from build123d import *

# Parameters (mm, degrees)
BOSS_EXTRUDE1_DEPTH = 5
FILLET1_R           = 2
FILLET2_R           = 1


with BuildPart() as part:
    # Sketch1 → Boss-Extrude1 (new body)
    with BuildSketch(Plane.XY):
        with BuildLine():
            Line((45.947382797642085, 2), (-124.5, 1.9999999999999962))
            Line((-124.5, 1.9999999999999962), (-124.5, 20.99999999999999))
            Line((-124.5, 20.99999999999999), (-109.6965869966638, 20.999999999999993))
            Line((-109.6965869966638, 20.999999999999993), (-109.6965869966638, 22.99999999999999))
            Line((-109.6965869966638, 22.99999999999999), (-126.5, 22.99999999999999))
            Line((-126.5, 22.99999999999999), (-126.5, -3.98e-15))
            Line((-126.5, -3.98e-15), (-96.00000000000003, -5.01e-15))
            ThreePointArc((-96.00000000000003, -1.3922e-13), (-91.91634498174992, -12.422936572760829), (-81.25831039658792, -19.999999999999993))
            Line((-81.25831039658792, -19.999999999999996), (-67.7416896034121, -19.999999999999996))
            ThreePointArc((-67.7416896034121, -20), (-59.22674645064795, -14.898875979359843), (-54.01801901082011, -6.449326782725662))
            ThreePointArc((-54.01801901082044, -6.449326782725638), (-49.745600463821845, -19.747926884371328), (-41.46929842095424, -31.000000000000007))
            Line((-41.46929842095423, -31), (-13.530701579045768, -31))
            ThreePointArc((-13.530701579045765, -31.000000000000004), (-5.5615533236631265, -20.33765705801185), (-1.1997684126617827, -7.76118245981885))
            ThreePointArc((-1.1997684126617756, -7.761182459818851), (1.6903832669508674, -16.34383705889386), (6.527542114603506, -24))
            Line((6.527542114603509, -24), (37.47245788539651, -24))
            ThreePointArc((37.47245788539651, -24), (44.12729350691807, -11.787963694678155), (45.947382797642085, 2))
        make_face()
        with BuildLine():
            ThreePointArc((-55.000000000000014, -3.1e-16), (-58.606442943263986, -11.117096597214955), (-68.05217786452643, -18))
            Line((-68.05217786452643, -18), (-80.94782213547359, -18))
            ThreePointArc((-80.94782213547359, -18.000000000000004), (-90.39355705673603, -11.117096597214955), (-94, -5.08e-15))
            Line((-94, -5.08e-15), (-55.00000000000001, -3.1e-16))
        make_face(mode=Mode.SUBTRACT)
        with BuildLine():
            ThreePointArc((-2.499999999999993, 0), (-5.579078670022007, -15.665382277262486), (-14.358195797467605, -28.999999999999996))
            Line((-14.358195797467618, -29), (-40.641804202532384, -29))
            ThreePointArc((-40.641804202532384, -29), (-49.420921329978, -15.665382277262491), (-52.500000000000014, 0))
            Line((-52.50000000000001, 0), (-2.5, 0))
        make_face(mode=Mode.SUBTRACT)
        with BuildLine():
            ThreePointArc((7.494737611193308, -21.999999999999993), (1.9251046025075595, -11.620790548201041), (0, 0))
            Line((0, 0), (44, 0))
            ThreePointArc((44, 0), (42.07489539749246, -11.620790548201052), (36.5052623888067, -22))
            Line((36.50526238880669, -22), (7.494737611193305, -21.999999999999986))
        make_face(mode=Mode.SUBTRACT)
    extrude(amount=BOSS_EXTRUDE1_DEPTH)

    # Fillet1
    # the kernel refuses this fillet: 2 mm, written as the material it adds along each edge
    with BuildSketch(Plane(origin=(7.494737611193306, -21.99999999999999, 0), x_dir=(-0.5991062369957058, 0.8006695428157894, 0), z_dir=(0, 0, 1))) as fillet1_piece_1:
        with BuildLine():
            CenterArc((1.0015491764552975, -1.9997957036664622), FILLET1_R, 89.18105145509278, 54.01303517716653)
            Line((-0.5997899091731567, -0.8015832296708748), (0, 0))
            ThreePointArc((0, 0), (0.5150674500576004, 0.00368108195627573), (1.030134900115199, -5e-17))
        make_face()
    extrude(amount=5)
    with BuildSketch(Plane(origin=(36.5052623888067, -22, 0), x_dir=(0.599106236995708, 0.8006695428157878, 0), z_dir=(0, 0, 1))) as fillet1_piece_2:
        with BuildLine():
            CenterArc((1.0015491764552726, 1.9997957036664615), FILLET1_R, 216.80591336773654, 54.01303517717065)
            Line((-0.5997899091732678, 0.8015832296709893), (0, 0))
            ThreePointArc((0, 0), (0.5150674500575887, -0.00368108195627645), (1.0301349001151745, 4e-17))
        make_face()
    extrude(amount=5)
    with BuildSketch(Plane(origin=(-1.1997684126617827, -7.7611824598188495, 0), x_dir=(-0.2559607440844839, -0.9666871766438806, 0), z_dir=(0, 0, 1))) as fillet1_piece_3:
        with BuildLine():
            CenterArc((7.006516264382127, 1.9937618524445377), FILLET1_R, 126.90247774602503, 138.57101311365483)
            ThreePointArc((5.80560665040515, 3.593079237786693), (2.9835854859434217, 1.6660138445939616), (0, 0))
            ThreePointArc((0, 0), (3.424337799359584, 0.13533600091225512), (6.84867559871917, -3e-17))
        make_face()
    extrude(amount=5)
    with BuildSketch(Plane(origin=(-14.358195797467612, -29, 0), x_dir=(0.6930946226970236, 0.720846616131664, 0), z_dir=(0, 0, 1))) as fillet1_piece_4:
        with BuildLine():
            CenterArc((0.8516205484031373, 1.9998888522074818), FILLET1_R, 223.8755770631898, 46.728475963226686)
            Line((-0.5900726838592292, 0.6136996068124346), (0, 0))
            ThreePointArc((0, 0), (0.4363527930685471, -0.00230019269212628), (0.8727055861370968, 1e-17))
        make_face()
    extrude(amount=5)
    with BuildSketch(Plane(origin=(-40.641804202532384, -29, 0), x_dir=(1, 0, 0), z_dir=(0, 0, 1))) as fillet1_piece_5:
        with BuildLine():
            CenterArc((0.8513594890752856, 2), FILLET1_R, 223.27152403673355, 46.72847596326642)
            ThreePointArc((-0.6048675489506863, 0.629086868644805), (-0.3040918605932177, 0.3129491831369968), (0, 0))
            Line((0, 0), (0.8513594890752856, 0))
        make_face()
    extrude(amount=5)
    with BuildSketch(Plane(origin=(-54.01801901082027, -6.449326782725651, 0), x_dir=(-0.4311999989802577, -0.9022563720359229, 0), z_dir=(0, 0, 1))) as fillet1_piece_6:
        with BuildLine():
            CenterArc((5.805573723556372, 1.9824143967569778), FILLET1_R, 131.58462794743895, 130.81175906112728)
            ThreePointArc((4.4781226039186794, 3.478366777340206), (2.2959426874147386, 1.6659530957609738), (0, 0))
            ThreePointArc((0, 0), (2.7704679671233965, 0.18410201579468238), (5.540935934246784, 1.2e-16))
        make_face()
    extrude(amount=5)
    with BuildSketch(Plane(origin=(-68.05217786452643, -18, 0), x_dir=(0.9475954690279733, 0.3194727329173106, 0), z_dir=(0, 0, 1))) as fillet1_piece_7:
        with BuildLine():
            CenterArc((0.3283173010527549, 1.9999162475023402), FILLET1_R, 251.36895898872925, 19.155393135414442)
            Line((-0.31062816478187977, 0.10472530944639823), (0, 0))
            ThreePointArc((0, 0), (0.17331019378626858, -0.00079304447276945), (0.34662038757253955, 0))
        make_face()
    extrude(amount=5)
    with BuildSketch(Plane(origin=(-80.94782213547359, -18.000000000000004, 0), x_dir=(1, 1.084e-14, 0), z_dir=(0, 0, 1))) as fillet1_piece_8:
        with BuildLine():
            CenterArc((0.32780672231424324, 2), FILLET1_R, 250.84460686458493, 19.155393135414442)
            ThreePointArc((-0.32845590873647146, 0.11073576250266372), (-0.1644813104532966, 0.05461639590219925), (0, 0))
            Line((0, 0), (0.3278067223142216, 0))
        make_face()
    extrude(amount=5)
    with BuildSketch(Plane(origin=(-96.00000000000003, -7.212e-14, 0), x_dir=(-1, 3.515e-14, 0), z_dir=(0, 0, 1))) as fillet1_piece_9:
        with BuildLine():
            CenterArc((1.912641367901373, 2), FILLET1_R, 185.00210139930942, 84.99789860069257)
            ThreePointArc((-0.07974163383531896, 1.82561544107731), (-0.01994490800398211, 0.9136780706116656), (0, 0))
            Line((0, 0), (1.9126413679014433, 0))
        make_face()
    extrude(amount=5)
    # the kernel refuses this fillet: 2 mm, written as the material it takes off along each edge
    with BuildSketch(Plane(origin=(45.947382797642085, 2.000000000000002, -5.001730056930275), x_dir=(0.026299501252087354, -0.9996541082964104, 0), z_dir=(0, 0, 1))) as fillet1_2_piece_1:
        with BuildLine():
            CenterArc((1.9480930202679383, -1.9993082165928209), FILLET1_R, 88.4929758152285, 89.9999999999682)
            Line((-0.05121519632485345, -1.9467092140875382), (0, 0))
            ThreePointArc((0, 0), (1.0003460113860576, 0.01315657596471321), (2.0006920227721112, 0))
        make_face()
    extrude(amount=15.003460113860552, mode=Mode.SUBTRACT)
    with BuildSketch(Plane(origin=(37.47245788539651, -24, -2.4841807127470568), x_dir=(-1, 0, 0), z_dir=(0, 0, 1))) as fillet1_2_piece_2:
        with BuildLine():
            CenterArc((0.9671954965845302, -2), FILLET1_R, 90, 52.37513808750745)
            ThreePointArc((-0.6168541298615224, -0.7790222029225369), (-0.3109710749573793, -0.3874966748050994), (0, 0))
            Line((0, 0), (0.9671954965845302, 0))
        make_face()
    extrude(amount=9.968361425494114, mode=Mode.SUBTRACT)
    with BuildSketch(Plane(origin=(6.527542114603495, -24, -2.484180712746931), x_dir=(-0.6207822630344314, 0.7839830239883068, 0), z_dir=(0, 0, 1))) as fillet1_2_piece_3:
        with BuildLine():
            CenterArc((0.9675482388101264, -1.9998293762732642), FILLET1_R, 89.2515799187701, 52.375138087411486)
            Line((-0.60041780916442, -0.7582648502017908), (0, 0))
            ThreePointArc((0, 0), (0.4968361425493905, 0.00324498101414436), (0.993672285098762, -4e-17))
        make_face()
    extrude(amount=9.96836142549386, mode=Mode.SUBTRACT)
    with BuildSketch(Plane(origin=(-13.53070157904575, -31, -2.118127681372563), x_dir=(-1, 0, 0), z_dir=(0, 0, 1))) as fillet1_2_piece_4:
        with BuildLine():
            CenterArc((0.8274942184199716, -2), FILLET1_R, 90, 45.520369910435846)
            ThreePointArc((-0.5995049670605166, -0.598688712441799), (-0.30121380534773223, -0.29788104203134225), (0, 0))
            Line((0, 0), (0.8274942184199716, 0))
        make_face()
    extrude(amount=9.236255362745126, mode=Mode.SUBTRACT)
    with BuildSketch(Plane(origin=(-41.469298420954246, -31, -2.118127681372557), x_dir=(1, 0, 0), z_dir=(0, 0, 1))) as fillet1_2_piece_5:
        with BuildLine():
            CenterArc((0.8274942184200782, 2), FILLET1_R, 224.47963008956205, 45.52036991043792)
            ThreePointArc((-0.5995049670604615, 0.5986887124418523), (-0.3012138053477287, 0.29788104203132804), (0, 0))
            Line((0, 0), (0.8274942184200782, 0))
        make_face()
    extrude(amount=9.236255362745114, mode=Mode.SUBTRACT)
    with BuildSketch(Plane(origin=(-67.7416896034121, -19.999999999999996, -0.8161799892839701), x_dir=(-1, 0, 0), z_dir=(0, 0, 1))) as fillet1_2_piece_6:
        with BuildLine():
            CenterArc((0.3104882611143438, -2), FILLET1_R, 90, 18.10668888712732)
            ThreePointArc((-0.3110865262256084, -0.09904108836006387), (-0.15573630283404327, -0.04891420940217017), (0, 0))
            Line((0, 0), (0.3104882611143438, 0))
        make_face()
    extrude(amount=6.632359978548406, mode=Mode.SUBTRACT)
    with BuildSketch(Plane(origin=(-81.25831039658793, -19.999999999999993, -0.8161799892839283), x_dir=(-0.9528735398862427, 0.3033677916072522, 0), z_dir=(0, 0, 1))) as fillet1_2_piece_7:
        with BuildLine():
            CenterArc((0.3108795347533545, -1.9999392178667164), FILLET1_R, 89.55330437229577, 18.106688887126865)
            Line((-0.2958560484611499, -0.09419213809423096), (0, 0))
            ThreePointArc((0, 0), (0.16323599785482176, 0.00063632240005913), (0.32647199570966445, 0))
        make_face()
    extrude(amount=6.632359978548333, mode=Mode.SUBTRACT)
    with BuildSketch(Plane(origin=(-109.6965869966638, 20.999999999999993, -5), x_dir=(-1, 0, 0), z_dir=(0, 0, 1)), Plane(origin=(-126.5, 22.99999999999999, -5), x_dir=(1, 0, 0), z_dir=(0, 0, 1))) as fillet1_2_piece_8:
        with BuildLine():
            CenterArc((FILLET1_R, -FILLET1_R), FILLET1_R, 90, 90)
            Line((0, -FILLET1_R), (0, 0))
            Line((0, 0), (FILLET1_R, 0))
        make_face()
    extrude(amount=15, mode=Mode.SUBTRACT)
    with BuildSketch(Plane(origin=(-109.6965869966638, 22.99999999999999, -5), x_dir=(0, -1, 0), z_dir=(0, 0, 1))) as fillet1_2_piece_9:
        with BuildLine():
            CenterArc((FILLET1_R, -FILLET1_R), FILLET1_R, 90, 90)
            Line((0, -FILLET1_R), (0, 0))
            Line((0, 0), (FILLET1_R, 0))
        make_face()
    extrude(amount=15, mode=Mode.SUBTRACT)
    with BuildSketch(Plane(origin=(-126.5, -3.55e-15, -5.000000000000001), x_dir=(0, 1, 0), z_dir=(0, 0, 1))) as fillet1_2_piece_10:
        with BuildLine():
            CenterArc((FILLET1_R, -FILLET1_R), FILLET1_R, 90, 90)
            Line((0, -FILLET1_R), (0, 0))
            Line((0, 0), (FILLET1_R, 0))
        make_face()
    extrude(amount=15, mode=Mode.SUBTRACT)

    # Fillet2
    # the kernel refuses this fillet: 1 mm, written as the material it takes off along each edge
    with BuildSketch(Plane(origin=(-109.96453618909511, 22, 9.999988187015607), x_dir=(-0.8660247217603869, -0.5000011812984491, 0), z_dir=(0, 0, -1))) as fillet2_piece_1:
        with BuildLine():
            CenterArc((1.4999964561018568, 0.8660260858068783), FILLET2_R, 120.0002344623185, 179.99968738357467)
            ThreePointArc((0.9999929122093405, 1.7320494435143525), (0.2679464643438091, 0.9999980028954786), (0, 0))
            ThreePointArc((0, 0), (0.9999976374012411, -0.26794782838624004), (1.999995274802482, 1.4e-16))
        make_face()
    extrude(amount=14.999976374031213, mode=Mode.SUBTRACT)


solid = part.part
The listing builds one solid part. Answer for the finished solid, in the listing's coordinates (mm). A direction names the side the tool comes from. Round coordinates to 2 decimals unless told otherwise and drop trailing zeros. Order: outer loops, then holes, each group sorted by start corner. A loop starts at its lowest first (then second) coordinate and runs counter-clockwise, first axis right, second up. Notation, with made-up numbers: (0, -27) -> (42, -27) arc R21 cw to (42, -11) -> close; hole circle Ø11 at (-39.5, 41.25). An arc over 180 degrees is marked (long way). Write each question's results on one line, items separated by ' | '. Start each with the question number.
Q1. Find section C-C (z = 2.6). Give the number of separate pieces and of enclosed holes in the cut face, then the cut area to 3 significant figures.
Q2. Straight lines are drawn through the part: probe 1 along Y at (x, z) = (14.5, 1.4); probe 2 along Y at (x, z) = (-73.5, 0.65); probe 3 along X at (y, z) = (-11.5, 0.7). For each, find the intervals that lie inside material, in ascending order. Write a range as from..to.
Q3. Find section A-A (x = 26.5). Determine the outline of the cut face in (y, z).
Q4. Which of the six approach directions +Z, -Z, +X, -X, +Y, -Y give full straight-line access (tool end or side, diameter ignored) to faces 5 (the flat face through (22, -22, 2)), 6 (the cylindrical face through (-7.13, -23.05, 2.46)), 7 (the flat face through (-53, -8, 0))?
Q5. Find section D-D (x = -45). Determine the outline of the cut face in (y, z).
Q6. The mould has two halves that part along X. Classify faces 1 (the flat face through (-118, 21, 2)), 2 (the cylindrical face through (-48.66, -21.74, 2.46)), 3 (the flat face through (-124.5, 11, 2)), 4 (the cylindrical face through (-91.57, -12.88, 2.46)): pulls with the +X half, pulls with the -X half, needs draft (parallel to the pull), parting line crosses it, or undercut.
Q7. Each of these flat-tipped pins is pushed along its axis until it touches: pin 1 (1.5 mm diameter, centred on x = 18, z = 3, fed in from -Y); pin 2 (10 mm diameter, centred on x = -87, y = -10.5, fed in from -Z); pin 3 (2.5 mm diameter, centred on x = -107.5, z = 3, fed in from -Y); pin 4 (2.5 mm diameter, centred on x = -31.5, z = 2, fed in from +Y). Where does it stop, or does it pass through?
Q8. Find section B-B (y = 6). Determine the outline of the cut face in (x, z).
Worked answers:
1) separate pieces: 1 | enclosed holes: 3 | area: 885 mm2
2) probe 1: y = -24..-22, 0..2 | probe 2: y = -20..-18, 0..2 | probe 3: x = -92.56..-90.11, -58.89..-56.44, -53.03..-50.87, -4.13..1.88, 42.12..44.22
3) outline: (-24, 0) -> (-22, 0) -> (-22, 5) -> (-24, 5) -> close; (0, 0) -> (2, 0) -> (2, 5) -> (0, 5) -> close
4) face 5: +Z, -Z | face 6: +Z, -Z, -Y | face 7: -Z, +X, -X, +Y, -Y
5) outline: (-27.1, 0) -> (-23.76, 0) -> (-23.76, 5) -> (-27.1, 5) -> close; (0, 0) -> (2, 0) -> (2, 5) -> (0, 5) -> close
6) face 1: needs draft | face 2: undercut | face 3: pulls with the +X half | face 4: pulls with the -X half
7) pin 1: stops at y = -24 | pin 2: stops at z = 0 | pin 3: stops at y = 0 | pin 4: stops at y = 2
8) outline: (-126.5, 0) -> (-124.5, 0) -> (-124.5, 5) -> (-126.5, 5) -> close
